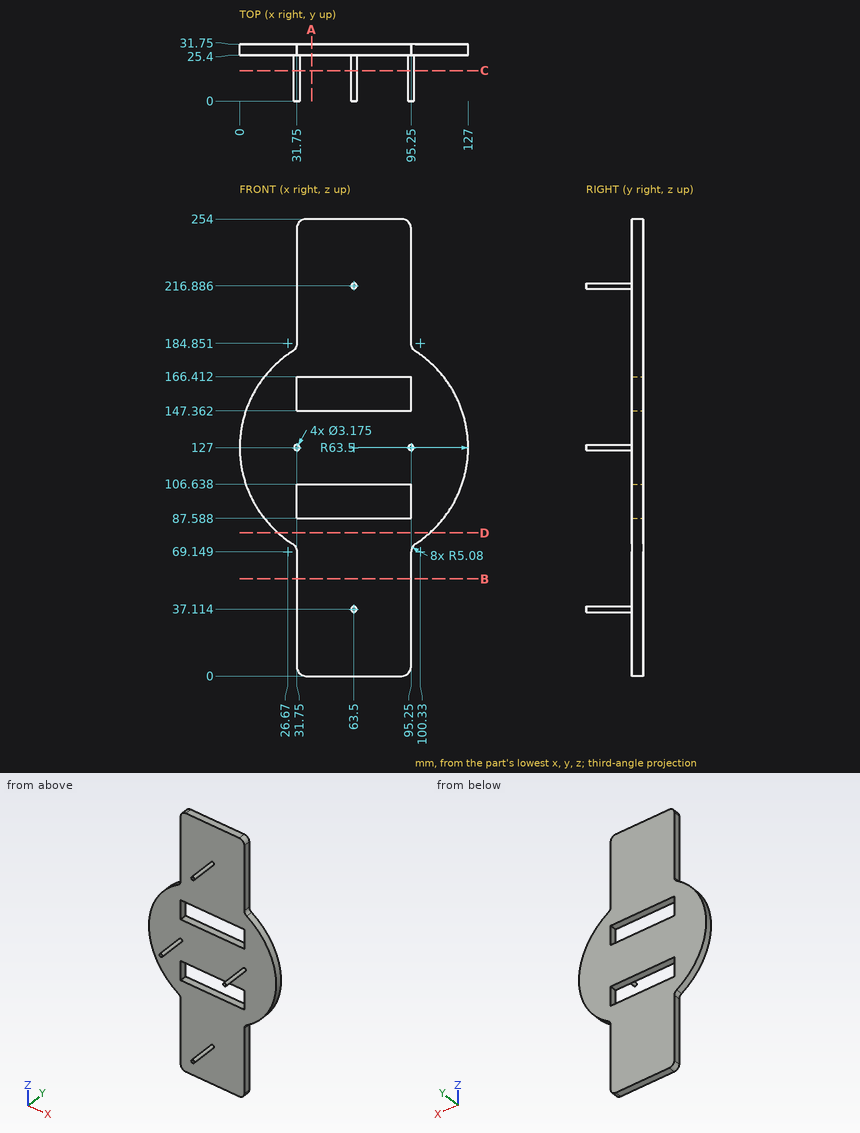
For this review, use the dimensioned drawing (mm, ordinates from the lowest corner) and the shaded views. Coordinates: 2 decimals unless noted, no trailing zeros. Loops run counter-clockwise (first coordinate to the right, second up) from the corner with the lowest first, then second, coordinate; pieces in that order, holes last. Notation, with made-up numbers: (9.25, 8.25) -> (22.25, 8.25) arc R29 ccw to (22.25, 30.25) -> close; hole circle Ø8 at (18.5, -19). An arc over 180 degrees is marked (long way). Use a Markdown table: item, result. Add a question column.
1. Add section A-A on x = 40. Write out the cut boundary in (y, z), plus the area to 3 significant figures.
2. Add section C-C on y = 17. Give the number of separate pieces and of enclosed holes in the cut face.
3. Add section B-B on z = 54. Write out the cut boundary in (x, y).
4. Add section D-D on z = 79.5. Write out the cut boundary in (x, y).
5. Clearance check with flat-ended pins moving along their axes: pin 1 Ø2 at (x, z) = (33.5, 207.5) entering from -Y; pin 2 Ø1 at (x, z) = (70, 149.5) entering from +Y (3 decimals); pin 3 Ø5 at (y, z) = (29.5, 221) entering from +X; pin 4 Ø1.9 at (y, z) = (28, 159.5) entering from +X. State where each tip first meets the part, or that it passes through.
6. To check wall thickness, follow line 1 (Z direction, x = 42.5, y = 29); line 2 (Y direction, x = 65.5, z = 21); line 3 (X direction, y = 10, z = 128). State the ranges of each line that lie inside material, in increasing order.
Returned:
| question | item | result |
|---|---|---|
| 1 | outline | (25.4, 0) -> (31.75, 0) -> (31.75, 87.59) -> (25.4, 87.59) -> close; (25.4, 106.64) -> (31.75, 106.64) -> (31.75, 147.36) -> (25.4, 147.36) -> close; (25.4, 166.41) -> (31.75, 166.41) -> (31.75, 254) -> (25.4, 254) -> close |
| 1 | area | 1,370 mm² |
| 2 | separate pieces | 4 |
| 2 | enclosed holes | 0 |
| 3 | outline | (31.75, 25.4) -> (95.25, 25.4) -> (95.25, 31.75) -> (31.75, 31.75) -> close |
| 4 | outline | (21.36, 25.4) -> (105.64, 25.4) -> (105.64, 31.75) -> (21.36, 31.75) -> close |
| 5 | pin 1 | stops at y = 25.4 |
| 5 | pin 2 | passes through |
| 5 | pin 3 | stops at x = 95.25 |
| 5 | pin 4 | stops at x = 118.61 |
| 6 | line 1 | z = 0 to 87.59, 106.64 to 147.36, 166.41 to 254 |
| 6 | line 2 | y = 25.4 to 31.75 |
| 6 | line 3 | x = 30.52 to 32.98, 94.02 to 96.48 |
